The model under review builds one solid part; all positions refer to its coordinate system, in mm. Face numbers are marked on the shaded views. A direction names the side the tool comes from. Coordinates: 2 decimals unless noted, no trailing zeros. Loops run counter-clockwise (first coordinate to the right, second up) from the corner with the lowest first, then second, coordinate; pieces in that order, holes last. Notation, with made-up numbers: (77.25, 68) - (86.25, 68) arc R3 cw to (86.25, 72) - close; hole circle Ø5 at (7, 33). An arc over 180 degrees is marked (long way). Answer in a Markdown table with one row per item. Add a question column.
(1) We need section B-B on x = -1.5. Write out the cut boundary in (y, z), plus the area to 3 significant figures.
(2) We need section C-C on y = 66.5. Write out the cut boundary in (x, z), plus the area to 3 significant figures.
(3) We need section D-D on x = 3.5. Write out the cut boundary in (y, z).
(4) For P1, Ø2.5, axis at y = -6.5, z = 2, coming from the +X side; P2, Ø5, axis at x = 6.5, y = -3, coming from the +Z side; P3, Ø4, axis at x = 5.5, z = -6, coming from the -Y side, all flat-tipped, find the tip position at first contact; note any pin that passes through.
(5) Mouldability with a two-part tool opening along X and no side actions: class the marked faces 1, 2, 3 and 4 as +X half, -X half, draft (parallel to the pull), parting line (faces both ways), or undercut.
(6) For line 1 along Y through (x, z) = (0, 2.5); line 2 along Y through (x, z) = (0.25, 7.25); line 3 along Y through (x, z) = (-7.75, -5.5), list the stretches that pass through material, from the lowest coordinate up.
(7) Machinability: for the marked faces 5 and 6, which of the approach directions +Z, -Z, +X, -X, +Y, -Y give a long, thin tool a straight path to every point of the face, cutting with its end or side? Answer none if there is none.
from build123d import *

# Parameters (mm, degrees)
SKETCH1_R           = 8
BOSS_EXTRUDE1_DEPTH = 80
SKETCH2_R           = 10
BOSS_EXTRUDE2_DEPTH = 3
SKETCH3_W           = 15
SKETCH3_H           = 10
BOSS_EXTRUDE3_DEPTH = 15
SKETCH4_R           = 5
CUT_EXTRUDE1_DEPTH  = 15
FILLET1_R           = 7.5


with BuildPart() as part:
    # Sketch1 → Boss-Extrude1 (new body)
    with BuildSketch(Plane(origin=(0, 0, 0), x_dir=(1, 0, 0), z_dir=(0, 1, 0))):
        with Locations(Location((0, 0, 0), (0, 0, 270))):
            Circle(SKETCH1_R)
    extrude(amount=BOSS_EXTRUDE1_DEPTH)

    # Sketch2 → Boss-Extrude2 (add)
    with BuildSketch(Plane.XZ):
        with Locations(Location((0, 0, 0), (0, 0, 270))):
            Circle(SKETCH2_R)
    extrude(amount=BOSS_EXTRUDE2_DEPTH)

    # Sketch3 → Boss-Extrude3 (add)
    with BuildSketch(Plane.XZ.offset(3)):
        Rectangle(SKETCH3_W, SKETCH3_H)
    extrude(amount=BOSS_EXTRUDE3_DEPTH)

    # Sketch4 → Cut-Extrude1 (cut)
    with BuildSketch(Plane(origin=(0, 0, -5), x_dir=(-1, 0, 0), z_dir=(0, 0, -1))):
        with Locations((0, -10.5)):
            Circle(SKETCH4_R)
    extrude(amount=-CUT_EXTRUDE1_DEPTH, mode=Mode.SUBTRACT)

    # Fillet1
    fillet1_edges = [part.edges().sort_by_distance(p)[0] for p in [
        (-7.5, -18, 0),
        (7.5, -18, 0),
    ]]
    fillet(fillet1_edges, radius=FILLET1_R - 0.0001)  # a hair under: the kernel refuses the full size


solid = part.part
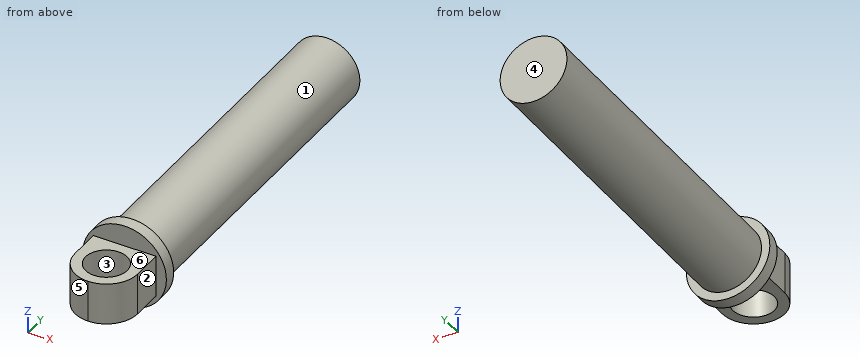
Outcome:
| question | item | result |
|---|---|---|
| 1 | outline | (-17.85, -5) - (-15.27, -5) - (-15.27, 5) - (-17.85, 5) - close; (-5.73, -5) - (-3, -5) - (-3, -9.89) - (0, -9.89) - (0, -7.86) - (80, -7.86) - (80, 7.86) - (0, 7.86) - (0, 9.89) - (-3, 9.89) - (-3, 5) - (-5.73, 5) - close |
| 1 | area | 1,370 mm² |
| 2 | outline | circle Ø16 at (0, 0) |
| 2 | area | 201 mm² |
| 3 | outline | (-17.13, -5) - (-14.07, -5) - (-14.07, 5) - (-17.13, 5) - close; (-6.93, -5) - (-3, -5) - (-3, -9.37) - (0, -9.37) - (0, -7.19) - (80, -7.19) - (80, 7.19) - (0, 7.19) - (0, 9.37) - (-3, 9.37) - (-3, 5) - (-6.93, 5) - close |
| 4 | P1 | x = 7.5 |
| 4 | P2 | z = 9.17 |
| 4 | P3 | y = -16.98 |
| 5 | face 1 | parting line |
| 5 | face 2 | +X half |
| 5 | face 3 | undercut |
| 5 | face 4 | draft |
| 6 | line 1 | -18 to -15.5, -5.5 to 80 |
| 6 | line 2 | -3 to 80 |
| 6 | line 3 | -3 to 0 |
| 7 | face 5 | +Z, -Z, -X, -Y |
| 7 | face 6 | +Z, +X, -X, -Y |
